```python
from build123d import *

# Parameters (mm, degrees)
SKETCH1_W           = 68.58
SKETCH1_H           = 53.34
BOSS_EXTRUDE1_DEPTH = 1.5
SKETCH2_W           = 12.7
SKETCH2_H           = 15.24
SKETCH2_W_2         = 3.39503639
SKETCH2_H_2         = 11.2855496
BOSS_EXTRUDE2_DEPTH = 5.08
SKETCH3_R           = 1.5875
CUT_EXTRUDE1_DEPTH  = 10.16
CUT_EXTRUDE2_DEPTH  = 2.5


with BuildPart() as part:
    # Sketch1 → Boss-Extrude1 (new body)
    with BuildSketch(Plane.XY):
        Rectangle(SKETCH1_W, SKETCH1_H)
    extrude(amount=BOSS_EXTRUDE1_DEPTH)

    # Sketch2 → Boss-Extrude2 (add)
    with BuildSketch(Plane.XY.offset(1.5)):
        with Locations((-34.29, 12.7)):
            Rectangle(SKETCH2_W, SKETCH2_H)
        with Locations((-34.29, -18.328779787)):
            Rectangle(SKETCH2_W_2, SKETCH2_H_2)
    extrude(amount=BOSS_EXTRUDE2_DEPTH)

    # Sketch3 → Cut-Extrude1 (cut)
    with BuildSketch(Plane.XY.offset(1.5)):
        with Locations((-19.05, 24.13)):
            Circle(SKETCH3_R)
        with Locations((-20.32, -24.13)):
            Circle(SKETCH3_R)
        with Locations((31.75, 8.89)):
            Circle(SKETCH3_R)
        with Locations((31.75, -19.05)):
            Circle(SKETCH3_R)
    extrude(amount=-CUT_EXTRUDE1_DEPTH, mode=Mode.SUBTRACT)

    # Sketch4 → Cut-Extrude2 (cut, through all)
    with BuildSketch(Plane.XY.offset(1.5)):
        Polygon((30.313159021, 26.67), (31.75, 25.233159021), (31.75, 13.012702255), (34.29, 11.115796447), (34.29, 26.67), align=None)
        Polygon((34.29, -23.181547096), (31.75, -25.078452904), (31.75, -26.67), (34.29, -26.67), align=None)
    extrude(amount=-CUT_EXTRUDE2_DEPTH, mode=Mode.SUBTRACT)


solid = part.part
```
Source: CAD feature listing. Evaluate the final solid. Frame: model axes, mm. A direction names the side the tool comes from. Coordinates: 2 decimals unless noted, no trailing zeros. Loops run counter-clockwise (first coordinate to the right, second up) from the corner with the lowest first, then second, coordinate; pieces in that order, holes last. Notation, with made-up numbers: M 49.5,62 L 73.5,62 A26 ccw 73.5,82 Z; hole C 37,28 d6. An arc over 180 degrees is marked long. Use a Markdown table: item, result. Add a question column.
Q1. First-contact query: pin 1 (1 mm diameter, centred on x = -35, z = 3, fed in from -Y); pin 2 (4 mm diameter, centred on x = 8.5, y = -14, fed in from +Z); pin 3 (1.6 mm diameter, centred on y = -25.5, z = 0.5, fed in from +X); pin 4 (1.9 mm diameter, centred on x = 31.75, y = 8.89, fed in from +Z). Flat tips, straight axial feed; report the tip coordinate or a pass-through.
Q2. Section query A-A, the plane y = 24.13. Return loops of the section in (x, z).
Q3. Draft query along Y for faces 1 (the flat face through (-35, -18, 1.5)), 2 (the flat face through (-2, -26.67, 1)), 3 (the flat face through (-34, 5.08, 4)). Return one class per face: pulls with the +Y half, pulls with the -Y half, needs draft (parallel to the pull), parting line crosses it, or undercut.
Q4. Section query C-C, the plane y = -14. Return loops of the section in (x, z).
Q5. Access query for faces 4 (the flat face through (-34, -12.686, 4)), 5 (the flat face through (-35.988, -18, 4)), 6 (the flat face through (-34.29, 0, 1)). Directions: +Z, -Z, +X, -X, +Y, -Y. A direction counts if a zero-diameter tool reaches every point of the face in a straight line with its end or side. Return the directions, or none.
Q6. Material intervals for L1, parallel to Y at x = -19.05, z = 0.8; L2, parallel to Z at x = 26, y = -21; L3, parallel to X at y = 10.5, z = 2.25, sorted ascending.
Q7. Section query D-D, the plane x = -24. Return loops of the section in (y, z), and give its area (3 significant figures).
Q8. Section query B-B, the plane z = 2.75. Return loops of the section in (x, y).
Result:
| question | item | result |
|---|---|---|
| 1 | pin 1 | stops at y = -23.97 |
| 1 | pin 2 | stops at z = 1.5 |
| 1 | pin 3 | stops at x = 32.26 |
| 1 | pin 4 | passes through |
| 2 | outline | M -34.29,0 L -20.64,0 L -20.64,1.5 L -34.29,1.5 Z; M -17.46,0 L 31.75,0 L 31.75,1.5 L -17.46,1.5 Z |
| 3 | face 1 | needs draft |
| 3 | face 2 | pulls with the -Y half |
| 3 | face 3 | undercut |
| 4 | outline | M -35.99,1.5 L -34.29,1.5 L -34.29,0 L 34.29,0 L 34.29,1.5 L -32.59,1.5 L -32.59,6.58 L -35.99,6.58 Z |
| 5 | face 4 | +Z, +X, -X |
| 5 | face 5 | +Z, -Z, -X, -Y |
| 5 | face 6 | -Z, -X, +Y, -Y |
| 6 | L1 | y = -26.67 to -25.08, -23.18 to 22.54, 25.72 to 26.67 |
| 6 | L2 | z = 0 to 1.5 |
| 6 | L3 | x = -40.64 to -27.94 |
| 7 | outline | M -26.67,0 L 26.67,0 L 26.67,1.5 L -26.67,1.5 Z |
| 7 | area | 80.0 mm2 |
| 8 | outline | M -40.64,5.08 L -27.94,5.08 L -27.94,20.32 L -40.64,20.32 Z; M -35.99,-23.97 L -32.59,-23.97 L -32.59,-12.69 L -35.99,-12.69 Z |
